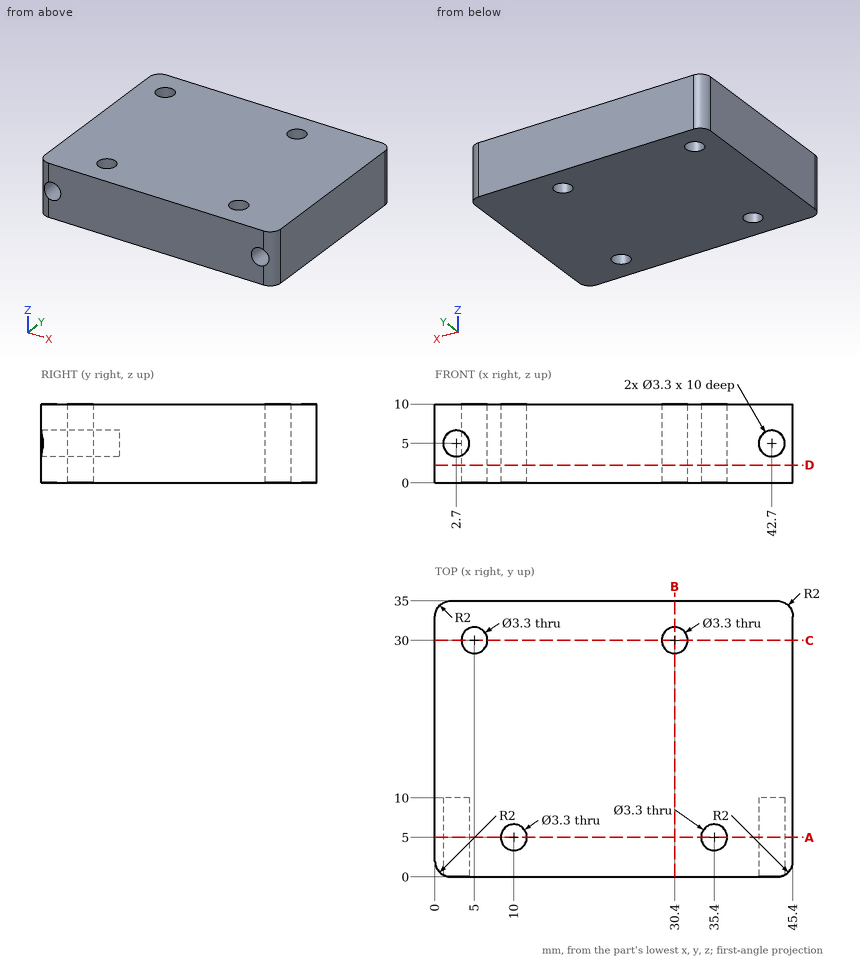
Answer from the drawing. Dimensions are ordinates in mm from the lowest x, y and z of the part. Give positions to 0.01 mm unless a question says otherwise; leave off trailing zeros. Loops run counter-clockwise (first coordinate to the right, second up) from the corner with the lowest first, then second, coordinate; pieces in that order, holes last. Notation, with made-up numbers: (49.25, 35) -> (72.25, 35) arc R4 cw to (72.25, 41) -> close; hole circle Ø11 at (-12.75, 51.25). An arc over 180 degrees is marked (long way). One line per question, with ' | ' between items. Start each with the question number.
1) Section C-C, the plane y = 30 is taken. Determine the outline of the cut face in (x, z).
2) Each of these flat-tipped pins is pushed along its axis until it touches: pin 1 (4 mm diameter, centred on x = 2.7, z = 5, fed in from -Y); pin 2 (1 mm diameter, centred on x = 2.5, z = 5, fed in from -Y). Where does it stop, or does it pass through?
3) Section B-B, the plane x = 30.4 is taken. Determine the outline of the cut face in (y, z), then the cut area to 3 significant figures.
4) Section A-A, the plane y = 5 is taken. Determine the outline of the cut face in (x, z), then the cut area to 3 significant figures.
5) Straight lines are drawn through the part: L1, parallel to X at y = 7.25, z = 5; L2, parallel to Y at x = 35.4, z = 5.5; L3, parallel to X at y = 3.5, z = 8.5. For each, find the intervals that lie inside material, in ascending order.
6) Section D-D, the plane z = 2.25 is taken. Determine the outline of the cut face in (x, y).
Resolved:
1) outline: (0, 0) -> (3.35, 0) -> (3.35, 10) -> (0, 10) -> close; (6.65, 0) -> (28.75, 0) -> (28.75, 10) -> (6.65, 10) -> close; (32.05, 0) -> (45.4, 0) -> (45.4, 10) -> (32.05, 10) -> close
2) pin 1: y = 0 | pin 2: y = 10
3) outline: (0, 0) -> (28.35, 0) -> (28.35, 10) -> (0, 10) -> close; (31.65, 0) -> (35, 0) -> (35, 10) -> (31.65, 10) -> close | area: 317 mm2
4) outline: (0, 0) -> (8.35, 0) -> (8.35, 10) -> (0, 10) -> close; (11.65, 0) -> (33.75, 0) -> (33.75, 10) -> (11.65, 10) -> close; (37.05, 0) -> (45.4, 0) -> (45.4, 10) -> (37.05, 10) -> close; hole circle Ø3.3 at (2.7, 5); hole circle Ø3.3 at (42.7, 5) | area: 371 mm2
5) L1: 0 to 1.05, 4.35 to 41.05, 44.35 to 45.4 | L2: 0 to 3.35, 6.65 to 35 | L3: 0 to 9.31, 10.69 to 34.71, 36.09 to 45.4
6) outline: (0, 2) arc R2 ccw to (2, 0) -> (43.4, 0) arc R2 ccw to (45.4, 2) -> (45.4, 33) arc R2 ccw to (43.4, 35) -> (2, 35) arc R2 ccw to (0, 33) -> close; hole circle Ø3.3 at (5, 30); hole circle Ø3.3 at (10, 5); hole circle Ø3.3 at (30.4, 30); hole circle Ø3.3 at (35.4, 5)
